For this review, use the dimensioned drawing (mm, ordinates from the lowest corner) and the shaded views. Give positions to 0.01 mm unless a question says otherwise; leave off trailing zeros. Order: outer loops, then holes, each group sorted by start corner. A loop starts at its lowest first (then second) coordinate and runs counter-clockwise, first axis right, second up.
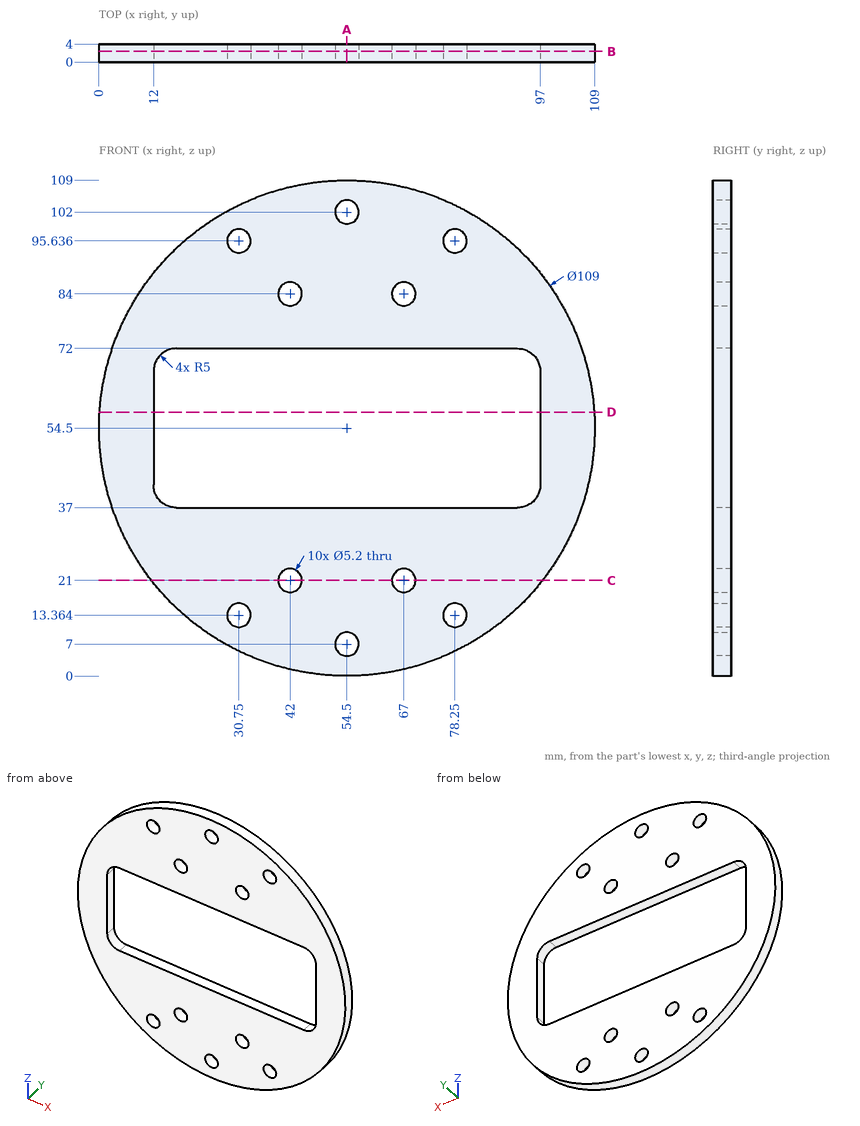
1. For pin 1 (2 mm diameter, centred on y = 2, z = 56, fed in from -X); pin 2 (1.2 mm diameter, centred on y = 1.5, z = 54, fed in from +X); pin 3 (1.2 mm diameter, centred on x = 42.5, y = 2.5, fed in from -Z), all flat-tipped, find the tip position at first contact; note any pin that passes through.
Recorded:
pin 1: stops at x = 0
pin 2: stops at x = 109
pin 3: stops at z = 1.21
2. Take a section at A-A (x = 54.5). State the section outline as (y, z) points, then the cut area to 3 significant figures.
Recorded:
outline: (0, 0) - (4, 0) - (4, 4.4) - (0, 4.4) - close; (0, 9.6) - (4, 9.6) - (4, 37) - (0, 37) - close; (0, 72) - (4, 72) - (4, 99.4) - (0, 99.4) - close; (0, 104.6) - (4, 104.6) - (4, 109) - (0, 109) - close
area: 254 mm2
3. Take a section at B-B (y = 2.4). State how many separate pieces and enclosed holes the cut face has, then the cut area to 3 significant figures.
Recorded:
separate pieces: 1
enclosed holes: 11
area: 6,170 mm2
4. Take a section at D-D (z = 58). State the section outline as (x, y) points.
Recorded:
outline: (0.11, 0) - (12, 0) - (12, 4) - (0.11, 4) - close; (97, 0) - (108.89, 0) - (108.89, 4) - (97, 4) - close
5. For line 1 along X through (y, z) = (1.1, 84) (1 decimal); line 2 along Z through (x, y) = (67, 1); line 3 along X through (y, z) = (2.6, 21), list the stretches that pass through material, from the lowest coordinate up.
Recorded:
line 1: x = 8.7 to 39.4, 44.6 to 64.4, 69.6 to 100.3
line 2: z = 1.45 to 18.4, 23.6 to 37, 72 to 81.4, 86.6 to 107.55
line 3: x = 11.51 to 39.4, 44.6 to 64.4, 69.6 to 97.49
6. Take a section at C-C (z = 21). State the section outline as (x, y) points, then the cut area to 3 significant figures.
Recorded:
outline: (11.51, 0) - (39.4, 0) - (39.4, 4) - (11.51, 4) - close; (44.6, 0) - (64.4, 0) - (64.4, 4) - (44.6, 4) - close; (69.6, 0) - (97.49, 0) - (97.49, 4) - (69.6, 4) - close
area: 302 mm2
